```python
from build123d import *

# Parameters (mm, degrees)
SKETCH1_R           = 4.1
BOSS_EXTRUDE1_DEPTH = 4
SKETCH2_R           = 4
CUT_EXTRUDE1_DEPTH  = 10
FILLET1_R           = 4
SKETCH3_R           = 4.1
CUT_EXTRUDE2_DEPTH  = 10
SKETCH4_R           = 4.1
BOSS_EXTRUDE3_DEPTH = 1.5
FILLET3_R           = 4


with BuildPart() as part:
    # Sketch1 → Boss-Extrude1 (new body)
    with BuildSketch(Plane(origin=(0, 0, 0), x_dir=(1, 0, 0), z_dir=(0, 1, 0))):
        Polygon((-8, 45), (-8, -45), (8, -45), (8, -8), (43, -8), (43, 8), (8, 8), (8, 45), align=None)
        with Locations(Location((0, 0, 0), (0, 0, 270))):
            Circle(SKETCH1_R, mode=Mode.SUBTRACT)
    extrude(amount=BOSS_EXTRUDE1_DEPTH)

    # Sketch2 → Cut-Extrude1 (cut)
    with BuildSketch(Plane(origin=(0, 4, 0), x_dir=(1, 0, 0), z_dir=(0, 1, 0))):
        with Locations(Location((0, -38, 0), (0, 0, 270))):
            Circle(SKETCH2_R)
    cut_extrude1 = extrude(amount=-CUT_EXTRUDE1_DEPTH, mode=Mode.SUBTRACT)

    # Mirror1: Cut-Extrude1 across plane
    add(cut_extrude1.mirror(Plane.XY), mode=Mode.SUBTRACT)

    # Fillet1
    fillet1_edges = [part.edges().sort_by_distance(p)[0] for p in [
        (43, 2, -8),
        (43, 2, 8),
        (8, 2, 8),
        (8, 2, 45),
        (-8, 2, 45),
        (-8, 2, -45),
        (8, 2, -45),
        (8, 2, -8),
    ]]
    fillet(fillet1_edges, radius=FILLET1_R)

    # Sketch3 → Cut-Extrude2 (cut)
    with BuildSketch(Plane(origin=(0, 4, 0), x_dir=(1, 0, 0), z_dir=(0, 1, 0))):
        with Locations(Location((35, 0, 0), (0, 0, 270))):
            Circle(SKETCH3_R)
    extrude(amount=-CUT_EXTRUDE2_DEPTH, mode=Mode.SUBTRACT)

    # Sketch4 → Boss-Extrude3 (add)
    with BuildSketch(Plane(origin=(0, 0, 0), x_dir=(1, 0, 0), z_dir=(0, 1, 0))):
        with BuildLine():
            Line((39, 8), (28, 8))
            Line((28, 8), (28, -8))
            Line((28, -8), (39, -8))
            ThreePointArc((39, -8), (41.828427125, -6.828427125), (43, -4))
            Line((43, -4), (43, 4))
            ThreePointArc((43, 4), (41.828427125, 6.828427125), (39, 8))
        make_face()
        with Locations(Location((35, 0, 0), (0, 0, 270))):
            Circle(SKETCH4_R, mode=Mode.SUBTRACT)
    extrude(amount=-BOSS_EXTRUDE3_DEPTH)

    # Fillet3
    # the kernel refuses this fillet: 4 mm, written as the material it adds along each edge
    with BuildSketch(Plane(origin=(28, 0, -8), x_dir=(0, -1, 0), z_dir=(0, 0, 1))) as fillet3_piece_1:
        with BuildLine():
            CenterArc((4, -3.122498999), FILLET3_R, 128.682187453, 51.317812547)
            Line((0, -3.122498999), (-0.08, -3.122498999))
            Line((-0.08, -3.122498999), (-0.08, 0))
            Line((-0.08, 0), (0, 0.08))
            ThreePointArc((0, 0.08), (0.75, 0.08), (1.45, 0.06244998))
            Line((1.45, 0.06244998), (1.5, 0))
        make_face()
    extrude(amount=16)


solid = part.part
```
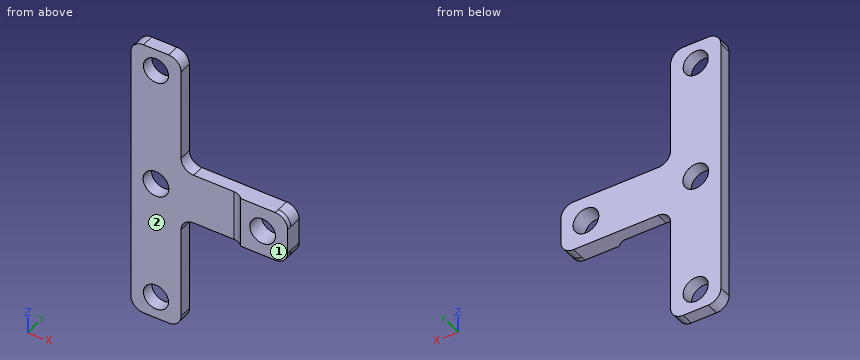
Here's how the part is built. I have some questions about the finished solid (model axes, mm). Face numbers are marked on the shaded views. A direction names the side the tool comes from. Coordinates: 2 decimals unless noted, no trailing zeros. Order: outer loops, then holes, each group sorted by start corner. A loop starts at its lowest first (then second) coordinate and runs counter-clockwise, first axis right, second up. Notation, with made-up numbers: (-22.5, -29) -> (17.5, -29) arc R24 ccw to (17.5, -17) -> close; hole circle Ø10 at (66.5, 38.25). An arc over 180 degrees is marked (long way). Return JSON: item names as keys, results as strings.
1) I'm going to push flat-ended pins straight in: P1, Ø10.5, axis at x = 0, z = -38, coming from the -Y side; P2, Ø13, axis at x = 35, z = 0, coming from the -Y side; P3, Ø1, axis at x = 6.5, y = 3, coming from the +Z side; P4, Ø1.7, axis at x = 31, y = 0, coming from the +Z side. Where does each tip first touch, or does it pass through?
Conclusion:
{"P1": "stops at y = 0", "P2": "stops at y = -1.5", "P3": "stops at z = 44.46", "P4": "stops at z = 8"}
2) If we section it at C-C on y = 2.9: List the corners of the cut face in (x, z) for me.
Conclusion:
{"outline": "(-8, -41) arc R4 ccw to (-4, -45) -> (4, -45) arc R4 ccw to (8, -41) -> (8, -12) arc R4 cw to (12, -8) -> (39, -8) arc R4 ccw to (43, -4) -> (43, 4) arc R4 ccw to (39, 8) -> (12, 8) arc R4 cw to (8, 12) -> (8, 41) arc R4 ccw to (4, 45) -> (-4, 45) arc R4 ccw to (-8, 41) -> close; hole circle Ø8.2 at (0, 0); hole circle Ø8 at (0, -38); hole circle Ø8 at (0, 38); hole circle Ø8.2 at (35, 0)"}
3) If I drill on probe 1 along X at (y, z) = (1.9, 0); probe 2 along X at (y, z) = (2.25, -38); probe 3 along Z at (x, y) = (2, 0.35), over which ranges is the centre line in solid material (lowest first)?
Conclusion:
{"probe 1": "x = -8 to -4.1, 4.1 to 30.9, 39.1 to 43", "probe 2": "x = -8 to -4, 4 to 8", "probe 3": "z = -45 to -41.46, -34.54 to -3.58, 3.58 to 34.54, 41.46 to 45"}
4) If we section it at A-A on z = -38: List the corners of the cut face in (x, y) for me.
Conclusion:
{"outline": "(-8, 0) -> (-4, 0) -> (-4, 4) -> (-8, 4) -> close; (4, 0) -> (8, 0) -> (8, 4) -> (4, 4) -> close"}
5) If we section it at B-B on x = 35: List the corners of the cut face in (y, z) for me.
Conclusion:
{"outline": "(-1.5, -8) -> (4, -8) -> (4, -4.1) -> (-1.5, -4.1) -> close; (-1.5, 4.1) -> (4, 4.1) -> (4, 8) -> (-1.5, 8) -> close"}
6) On a 3-axis mill with a long thin cutter (end or side, diameter ignored), from which of +Z, -Z, +X, -X, +Y, -Y can I reach the whole of each face in a straight line? I mean the marked faces 1 and 2. Say none if no direction works.
Conclusion:
{"face 1": "+Z, -Z, +X, -X, -Y", "face 2": "+Z, -Z, -X, -Y"}
7) If we section it at D-D on x = 0: List the corners of the cut face in (y, z) for me.
Conclusion:
{"outline": "(0, -45) -> (4, -45) -> (4, -42) -> (0, -42) -> close; (0, -34) -> (4, -34) -> (4, -4.1) -> (0, -4.1) -> close; (0, 4.1) -> (4, 4.1) -> (4, 34) -> (0, 34) -> close; (0, 42) -> (4, 42) -> (4, 45) -> (0, 45) -> close"}
